Source: CAD feature listing. Evaluate the final solid. Frame: model axes, mm. A direction names the side the tool comes from. Round coordinates to 2 decimals unless told otherwise and drop trailing zeros. Loops run counter-clockwise (first coordinate to the right, second up) from the corner with the lowest first, then second, coordinate; pieces in that order, holes last.
(1) Set-up query: faces 4 (the cylindrical face through (-87.648, 4.923, 11.076)), 5 (the flat face through (-1, 35.56, 39)). Return all of +Z, -Z, +X, -X, +Y, -Y with unobstructed straight access to the full face (end or side cutting, diameter ignored); none if empty.
(2) First-contact query: pin 1 Ø2.5 at (y, z) = (11.97, 9.47) entering from +X; pin 2 Ø12 at (x, y) = (-35, 25) entering from +Z. Flat tips, straight axial feed; report the tip coordinate or a pass-through.
(3) Section A-A, the plane y = 0. Return the cut outline in (x, z).
(4) Section C-C, the plane x = -28. Return the cut outline in (y, z), plus the area to 3 significant figures.
(5) Material intervals for probe 1 along Y at (x, z) = (3.5, 52); probe 2 along X at (y, z) = (-1, 58.5); probe 3 along Z at (x, y) = (-4.5, -16), sorted ascending.
(6) Mould query, pull axis Y, two halves, no side actions, for faces 1 (the cylindrical face through (-87.65, -5.7, 11.36)), 2 (the flat face through (0, 37, 76.2)), 3 (the flat face through (-1, 38.1, 38)). Classes: pulls with the +Y half, pulls with the -Y half, needs draft (parallel to the pull), parting line crosses it, or undercut.
(7) Section B-B, the plane z = 18.5. Return the cut outline in (x, y).
```python
from build123d import *

# Parameters (mm, degrees)
F0_W     = 177.8
F0_H     = 76.2
F1_DEPTH = 76.2
F3_T     = -2.54
F4_D     = 3.81


with BuildPart() as f1:
    # F0 (on Top) → F1 (new body)
    with BuildSketch(Plane.XY):
        Rectangle(F0_W, F0_H)
    extrude(amount=F1_DEPTH)

    # F3
    f3_openings = [f1.faces().sort_by_distance(p)[0] for p in [
        (0, 0, 76.2),
    ]]
    offset(amount=F3_T, openings=f3_openings)

    # F4 (through all)
    with Locations(Plane.YZ.offset(88.9)):
        with Locations((-30.918453, 9.469561), (-24.460413, 9.469561), (-18.648177, 9.469561), (-5.947364, 9.469561), (-11.974867, 9.469561), (0, 9.469561), (5.947364, 9.469561), (11.974867, 9.469561), (18.648177, 9.469561), (24.460413, 9.469561), (31.509273, 9.469561)):
            Hole(F4_D / 2)


solid = f1.part
```
Output values:
1. face 4: +X, -X
1. face 5: +Z
2. pin 1: passes through
2. pin 2: stops at z = 2.54
3. outline: (-88.9, 0) - (88.9, 0) - (88.9, 7.56) - (86.36, 7.56) - (86.36, 2.54) - (-86.36, 2.54) - (-86.36, 7.56) - (-88.9, 7.56) - close; (-88.9, 11.37) - (-86.36, 11.37) - (-86.36, 76.2) - (-88.9, 76.2) - close; (86.36, 11.37) - (88.9, 11.37) - (88.9, 76.2) - (86.36, 76.2) - close
4. outline: (-38.1, 0) - (38.1, 0) - (38.1, 76.2) - (35.56, 76.2) - (35.56, 2.54) - (-35.56, 2.54) - (-35.56, 76.2) - (-38.1, 76.2) - close
4. area: 568 mm2
5. probe 1: y = -38.1 to -35.56, 35.56 to 38.1
5. probe 2: x = -88.9 to -86.36, 86.36 to 88.9
5. probe 3: z = 0 to 2.54
6. face 1: undercut
6. face 2: needs draft
6. face 3: pulls with the +Y half
7. outline: (-88.9, -38.1) - (88.9, -38.1) - (88.9, 38.1) - (-88.9, 38.1) - close; hole (-86.36, -35.56) - (86.36, -35.56) - (86.36, 35.56) - (-86.36, 35.56) - close
